```python
from build123d import *

# Parameters (mm, degrees)
SKETCH1_R               = 45
BOSS_EXTRUDE1_DEPTH     = 80
SKETCH2_W               = 68.94399988
SKETCH2_H               = 120
BOSS_EXTRUDE2_DEPTH     = 80
CUT_EXTRUDE1_START      = -70
SKETCH3_R               = 40.5
CUT_EXTRUDE1_DEPTH      = 70
CUT_EXTRUDE2_REACH      = 176.939
SKETCH4_R               = 10
CUT_EXTRUDE3_REACH      = 176.939
CUT_EXTRUDE4_REACH      = 200.874
CUT_EXTRUDE4_END_RADIUS = 45
SKETCH6_W               = 58.94399988
SKETCH6_H               = 70
CUT_EXTRUDE5_REACH      = 200.874
CUT_EXTRUDE5_END_RADIUS = 45
SKETCH7_W               = 48.94399988
SKETCH7_H               = 5
CUT_EXTRUDE6_START      = -103.925442
SKETCH8_W               = 5
SKETCH8_H               = 60
CUT_EXTRUDE6_DEPTH      = 103.925442
SKETCH9_W               = 65
SKETCH9_H               = 60
CUT_EXTRUDE7_DEPTH      = 60
SKETCH11_W              = 68.94399988
SKETCH11_H              = 80
BOSS_EXTRUDE3_DEPTH     = 15
SKETCH12_W              = 15
SKETCH12_H              = 5
BOSS_EXTRUDE4_DEPTH     = 15
FILLET1_R               = 7.5
CUT_EXTRUDE8_REACH      = 180.061
SKETCH13_R              = 3.5
FILLET2_R               = 5
FILLET3_R               = 5
SKETCH15_R              = 15
BOSS_EXTRUDE5_DEPTH     = 4.5
SKETCH16_R              = 11.25
CUT_EXTRUDE9_DEPTH      = 7.5
SKETCH17_R              = 3.25
CUT_EXTRUDE10_DEPTH     = 15


with BuildPart() as part:
    # Sketch1 → Boss-Extrude1 (new body)
    with BuildSketch(Plane.XY):
        Circle(SKETCH1_R)
    extrude(amount=BOSS_EXTRUDE1_DEPTH)

    # Sketch2 → Boss-Extrude2 (add)
    with BuildSketch(Plane(origin=(0, 0, 0), x_dir=(-1, 0, 0), z_dir=(0, 0, -1))):
        with Locations((0, -88.925442436)):
            Rectangle(SKETCH2_W, SKETCH2_H)
    extrude(amount=-BOSS_EXTRUDE2_DEPTH)

    # Sketch3 → Cut-Extrude1 (cut)
    with BuildSketch(Plane(origin=(0, 0, 5), x_dir=(-1, 0, 0), z_dir=(0, 0, -1)).offset(CUT_EXTRUDE1_START)):
        Circle(SKETCH3_R)
    extrude(amount=CUT_EXTRUDE1_DEPTH, mode=Mode.SUBTRACT)

    # Cut-Extrude2: up to this face of the body (flat: up to its plane)
    cut_extrude2_end = Plane(part.part.faces().sort_by_distance((0, -51.092470511, 80))[0])
    # Sketch4 → Cut-Extrude2 (cut, up to the picked face)
    with BuildSketch(Plane(origin=(0, 0, 0), x_dir=(-1, 0, 0), z_dir=(0, 0, -1)), mode=Mode.PRIVATE) as cut_extrude2_sk1:
        Circle(SKETCH4_R)
    cut_extrude2_tool1 = split(extrude(cut_extrude2_sk1.sketch, amount=-CUT_EXTRUDE2_REACH, mode=Mode.PRIVATE), bisect_by=cut_extrude2_end, keep=Keep.BOTH, mode=Mode.PRIVATE)
    add(cut_extrude2_tool1.solids().sort_by(Axis((0, 0, 0), (0, 0, 1)))[0], mode=Mode.SUBTRACT)

    # Cut-Extrude3: up to this face of the body (flat: up to its plane)
    cut_extrude3_end = Plane(part.part.faces().sort_by_distance((0, -52.276987432, 80))[0])
    # Sketch5 → Cut-Extrude3 (cut, up to the picked face)
    with BuildSketch(Plane(origin=(0, 0, 0), x_dir=(-1, 0, 0), z_dir=(0, 0, -1)), mode=Mode.PRIVATE) as cut_extrude3_sk1:
        with BuildLine():
            Line((-26.562960223, 7.11752374), (-43.466662183, 11.64685703))
            ThreePointArc((-43.466662183, 11.64685703), (17.220754456, 41.574578963), (38.97114317, -22.5))
            Line((38.97114317, -22.5), (23.815698604, -13.75))
            ThreePointArc((23.815698604, -13.75), (10.52379439, 25.406687144), (-26.562960223, 7.11752374))
        make_face()
    cut_extrude3_tool1 = split(extrude(cut_extrude3_sk1.sketch, amount=-CUT_EXTRUDE3_REACH, mode=Mode.PRIVATE), bisect_by=cut_extrude3_end, keep=Keep.BOTH, mode=Mode.PRIVATE)
    add(cut_extrude3_tool1.solids().sort_by(Axis((-31.949807, -17.161312, 0), (0, 0, 1)))[0], mode=Mode.SUBTRACT)

    # Cut-Extrude4: up to this cylinder (the profile starts outside it)
    cut_extrude4_end = Plane(origin=(0, 0, 40), z_dir=(0, 0, -1)) * Cylinder(CUT_EXTRUDE4_END_RADIUS, 492.748, mode=Mode.PRIVATE)
    # Sketch6 → Cut-Extrude4 (cut, up to the surface)
    with BuildSketch(Plane.XZ.offset(148.925442436), mode=Mode.PRIVATE) as cut_extrude4_sk1:
        with Locations((0, 40)):
            Rectangle(SKETCH6_W, SKETCH6_H)
    cut_extrude4_tool1 = extrude(cut_extrude4_sk1.sketch, amount=-CUT_EXTRUDE4_REACH, mode=Mode.PRIVATE) - cut_extrude4_end
    add(cut_extrude4_tool1.solids().sort_by_distance((0, -148.925442, 40))[0], mode=Mode.SUBTRACT)

    # Cut-Extrude5: up to this cylinder (the profile starts outside it)
    cut_extrude5_end = Plane(origin=(0, 0, 40), z_dir=(0, 0, -1)) * Cylinder(CUT_EXTRUDE5_END_RADIUS, 567.748, mode=Mode.PRIVATE)
    # Sketch7 → Cut-Extrude5 (cut, up to the surface)
    with BuildSketch(Plane.XZ.offset(148.925442436), mode=Mode.PRIVATE) as cut_extrude5_sk1:
        with Locations((0, 77.5)):
            Rectangle(SKETCH7_W, SKETCH7_H)
    cut_extrude5_tool1 = extrude(cut_extrude5_sk1.sketch, amount=-CUT_EXTRUDE5_REACH, mode=Mode.PRIVATE) - cut_extrude5_end
    add(cut_extrude5_tool1.solids().sort_by_distance((0, -148.925442, 77.5))[0], mode=Mode.SUBTRACT)
    # Sketch7 → Cut-Extrude5 (cut, up to the surface)
    with BuildSketch(Plane.XZ.offset(148.925442436), mode=Mode.PRIVATE) as cut_extrude5_sk2:
        with Locations((0, 2.5)):
            Rectangle(SKETCH7_W, SKETCH7_H)
    cut_extrude5_tool2 = extrude(cut_extrude5_sk2.sketch, amount=-CUT_EXTRUDE5_REACH, mode=Mode.PRIVATE) - cut_extrude5_end
    add(cut_extrude5_tool2.solids().sort_by_distance((0, -148.925442, 2.5))[0], mode=Mode.SUBTRACT)

    # Sketch8 → Cut-Extrude6 (cut)
    with BuildSketch(Plane.XZ.offset(148.925442436).offset(CUT_EXTRUDE6_START)):
        with Locations((31.97199994, 40)):
            Rectangle(SKETCH8_W, SKETCH8_H)
    extrude(amount=CUT_EXTRUDE6_DEPTH, mode=Mode.SUBTRACT)

    # Sketch9 → Cut-Extrude7 (cut)
    with BuildSketch(Plane(origin=(0, -20.25, 0), x_dir=(1, 0, 0), z_dir=(0, 1, 0))):
        with Locations((-6.47114317, -40)):
            Rectangle(SKETCH9_W, SKETCH9_H)
    extrude(amount=-CUT_EXTRUDE7_DEPTH, mode=Mode.SUBTRACT)

    # Sketch11 → Boss-Extrude3 (add)
    with BuildSketch(Plane.XZ.offset(148.925442436)):
        with Locations((0, 40)):
            Rectangle(SKETCH11_W, SKETCH11_H)
    extrude(amount=BOSS_EXTRUDE3_DEPTH)

    # Sketch12 → Boss-Extrude4 (add)
    with BuildSketch(Plane(origin=(0, -148.925442436, 0), x_dir=(1, 0, 0), z_dir=(0, 1, 0))):
        with Locations((16.97199994, -29.5)):
            Rectangle(SKETCH12_W, SKETCH12_H)
        with Locations((16.97199994, -50.5)):
            Rectangle(SKETCH12_W, SKETCH12_H)
    extrude(amount=BOSS_EXTRUDE4_DEPTH)

    # Fillet1
    fillet1_edges = [part.edges().sort_by_distance(p)[0] for p in [
        (24.47199994, -133.925442436, 50.5),
        (9.47199994, -133.925442436, 50.5),
        (24.47199994, -133.925442436, 29.5),
        (9.47199994, -133.925442436, 29.5),
    ]]
    fillet(fillet1_edges, radius=FILLET1_R - 0.0001)  # a hair under: the kernel refuses the full size

    # Cut-Extrude8: up to this face of the body (flat: up to its plane)
    cut_extrude8_end = Plane(part.part.faces().sort_by_distance((16.97199994, -142.125548149, 53))[0])
    # Sketch13 → Cut-Extrude8 (cut, up to the picked face)
    with BuildSketch(Plane(origin=(0, 0, 27), x_dir=(-1, 0, 0), z_dir=(0, 0, -1)), mode=Mode.PRIVATE) as cut_extrude8_sk1:
        with Locations((-16.97199994, -141.425442436)):
            Circle(SKETCH13_R)
    cut_extrude8_tool1 = split(extrude(cut_extrude8_sk1.sketch, amount=-CUT_EXTRUDE8_REACH, mode=Mode.PRIVATE), bisect_by=cut_extrude8_end, keep=Keep.BOTH, mode=Mode.PRIVATE)
    add(cut_extrude8_tool1.solids().sort_by(Axis((16.972, -141.425442, 27), (0, 0, 1)))[0], mode=Mode.SUBTRACT)

    # Fillet2
    fillet2_edges = [part.edges().sort_by_distance(p)[0] for p in [
        (34.47199994, -96.425442436, 0),
        (-34.47199994, -96.425442436, 0),
        (34.47199994, -96.425442436, 80),
        (-34.47199994, -96.425442436, 80),
        (-34.47199994, -163.925442436, 40),
        (0, -163.925442436, 0),
        (34.47199994, -163.925442436, 40),
        (0, -163.925442436, 80),
    ]]
    fillet(fillet2_edges, radius=FILLET2_R)

    # Fillet3
    fillet3_edges = [part.edges().sort_by_distance(p)[0] for p in [
        (26.02885683, -33.868240693, 10),
        (-31.97199994, -80.25, 10),
        (-31.97199994, -80.25, 70),
        (26.02885683, -33.868240693, 70),
    ]]
    fillet(fillet3_edges, radius=FILLET3_R)

    # Sketch15 → Boss-Extrude5 (add)
    with BuildSketch(Plane(origin=(0, 0, 0), x_dir=(-1, 0, 0), z_dir=(0, 0, -1))):
        with Locations(Location((0, 0, 0), (0, 0, 180))):
            Circle(SKETCH15_R)
    boss_extrude5 = extrude(amount=BOSS_EXTRUDE5_DEPTH)

    # Mirror1: Boss-Extrude5 across plane
    add(boss_extrude5.mirror(Plane.XY.offset(40)))

    # Sketch16 → Cut-Extrude9 (cut)
    with BuildSketch(Plane(origin=(0, 0, -4.5), x_dir=(-1, 0, 0), z_dir=(0, 0, -1))):
        Circle(SKETCH16_R)
    cut_extrude9 = extrude(amount=-CUT_EXTRUDE9_DEPTH, mode=Mode.SUBTRACT)

    # Mirror2: Cut-Extrude9 across plane
    add(cut_extrude9.mirror(Plane.XY.offset(40)), mode=Mode.SUBTRACT)

    # Sketch17 → Cut-Extrude10 (cut)
    with BuildSketch(Plane.XZ.offset(163.925442436)):
        with Locations(Location((-19.955, 59.955, 0), (0, 0, 270))):
            Circle(SKETCH17_R)
        with Locations(Location((19.955, 59.955, 0), (0, 0, 270))):
            Circle(SKETCH17_R)
        with Locations(Location((19.955, 20.045, 0), (0, 0, 270))):
            Circle(SKETCH17_R)
        with Locations(Location((-19.955, 20.045, 0), (0, 0, 270))):
            Circle(SKETCH17_R)
    extrude(amount=-CUT_EXTRUDE10_DEPTH, mode=Mode.SUBTRACT)


solid = part.part
```
Design review of the part built by this model. Coordinates are the model's own, in mm. A direction names the side the tool comes from. Coordinates: 2 decimals unless noted, no trailing zeros. Write each loop counter-clockwise with the first axis right and the second up, starting at its lowest first coordinate (ties: lowest second). Pieces come first, ordered by that corner, then holes.
1) Add section D-D (z = 59.5). Write out the cut boundary in (x, y), plus the area to 3 significant figures.
2) Mouldability with a two-part tool opening along Z and no side actions: class faces 1 (the flat face through (-29.472, -105, 40)), 2 (the flat face through (2.8, -44.6, 0)), 3 (the cylindrical face through (11.61, -136.18, 50.46)), 4 (the flat face through (27, -92, 5)) as +Z half, -Z half, draft (parallel to the pull), parting line (faces both ways), or undercut.
3) Machinability: for faces 5 (the flat face through (-32, -80.25, 40)), 6 (the flat face through (9.472, -145, 30)), 7 (the flat face through (19, -145, 27)), 8 (the flat face through (26.029, -34, 40)), 9 (the flat face through (27, -92, 75)), which of the approach directions +Z, -Z, +X, -X, +Y, -Y give a long, thin tool a straight path to every point of the face, cutting with its end or side? Answer none if there is none.
4) Add section B-B (y = 0). State how many separate pieces and enclosed holes the cut face has, plus the area to 4 significant figures.
5) To check wall thickness, follow L1, parallel to Z at x = -27, y = -60; L2, parallel to Z at x = 0, y = 14.5; L3, parallel to Y at x = 26, z = 11.5. State the ranges of each line that lie inside material, in increasing order.
6) Insertion check: pin 1 (5 mm diameter, centred on y = -109, z = 10, fed in from -X); pin 2 (4 mm diameter, centred on x = -27, y = -105, fed in from -Z); pin 3 (5 mm diameter, centred on x = 10.5, z = 37.5, fed in from +Y). Each pin has a flat end and moves straight along its axis. Give the tip position at first contact, or say it passes through.
7) Add section A-A (z = 8). Write out the cut boundary in (x, y), plus the area to 3 significant figures.
Check result:
1. outline: (-34.47, -158.93) arc R5 ccw to (-29.47, -163.93) - (-23.17, -163.93) - (-23.17, -148.93) - (-29.47, -148.93) - (-29.47, -80.25) - (-34.47, -80.25) - close; (-16.74, -163.93) - (16.74, -163.93) - (16.74, -148.93) - (-16.74, -148.93) - close; (23.17, -163.93) - (29.47, -163.93) arc R5 ccw to (34.47, -158.93) - (34.47, -148.93) - (23.17, -148.93) - close; (26.03, -36.71) arc R45 ccw to (29.47, -34.01) - (29.47, -45) - (34.47, -45) - (34.47, -28.93) arc R45 ccw to (43.47, 11.65) - (39.12, 10.48) arc R40.5 cw to (26.03, -31.03) - close
1. area: 1,470 mm2
2. face 1: undercut
2. face 2: -Z half
2. face 3: draft
2. face 4: undercut
3. face 5: +X, -X, +Y
3. face 6: +Z, -Z, +Y
3. face 7: -Z, +X, +Y
3. face 8: -X, +Y
3. face 9: none
4. separate pieces: 3
4. enclosed holes: 0
4. area: 892.5 mm2
5. L1: z = 0 to 5, 75 to 80
5. L2: z = -4.5 to 5, 75 to 84.5
5. L3: y = -163.93 to -148.93, -36.73 to -31.05
6. pin 1: stops at x = -34.47
6. pin 2: stops at z = 0
6. pin 3: stops at y = -148.93
7. outline: (-38.97, -22.5) arc R45 ccw to (-34.47, -28.93) - (-34.47, -158.93) arc R5 ccw to (-29.47, -163.93) - (29.47, -163.93) arc R5 ccw to (34.47, -158.93) - (34.47, -28.93) arc R45 ccw to (43.47, 11.65) - (39.12, 10.48) arc R40.5 cw to (-35.07, -20.25) - close; hole (-29.47, -148.93) - (29.47, -148.93) - (29.47, -34.01) arc R45 cw to (-29.47, -34.01) - close
7. area: 2,750 mm2
